CAD build for the part. Positions are in the model's coordinates, mm. Face numbers are marked on the shaded views. A direction names the side the tool comes from. Give positions to 0.01 mm unless a question says otherwise; leave off trailing zeros. Loops run counter-clockwise (first coordinate to the right, second up) from the corner with the lowest first, then second, coordinate; pieces in that order, holes last. Notation, with made-up numbers: M -9,45 L 50,45 A23 ccw 50,68 Z; hole C 35,70 d1. An arc over 180 degrees is marked long. Answer as CSV lines item,"result".
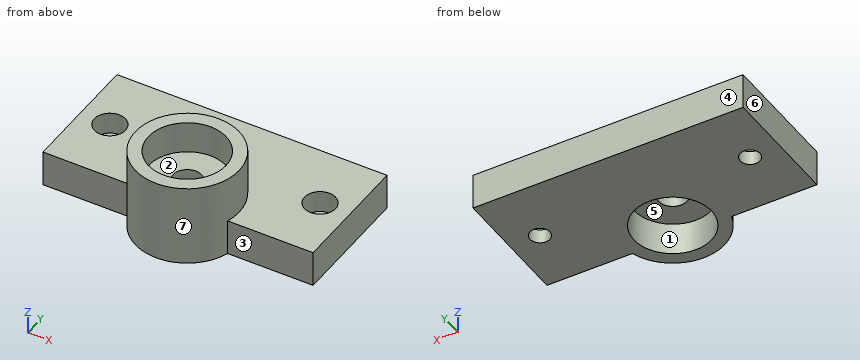
from build123d import *

# Parameters (mm, degrees)
F0_R     = 17.765
F0_R_2   = 13.28
F1_DEPTH = 27.96
F2_START = 11.06
F0_R_3   = 4.91
F2_DEPTH = 5.99
F3_R     = 5.32
F4_DEPTH = 12.28
F3_R_2   = 3.41
F5_DEPTH = 4.8


with BuildPart() as f1:
    # F0 (on Top) → F1 (new body)
    with BuildSketch(Plane.XY):
        Circle(F0_R)
        Circle(F0_R_2, mode=Mode.SUBTRACT)
    extrude(amount=F1_DEPTH)

    # F0 (on Top) → F2 (join)
    with BuildSketch(Plane.XY.offset(F2_START)):
        Circle(F0_R_2)
        Circle(F0_R_3, mode=Mode.SUBTRACT)
    extrude(amount=F2_DEPTH)

    # F3 (on Top) → F4 (join)
    with BuildSketch(Plane.XY):
        with BuildLine():
            Line((46.155, -5.28), (46.155, 37.06))
            Line((46.155, 37.06), (-46.155, 37.06))
            Line((-46.155, 37.06), (-46.155, -5.28))
            Line((-46.155, -5.28), (-12.1852369694, -5.28))
            ThreePointArc((-12.1852369694, -5.28), (-2.6961503154, 13.0034292968), (13.28, 0))
            ThreePointArc((13.28, 0), (13.0034292968, -2.6961503154), (12.1852369694, -5.28))
            Line((12.1852369694, -5.28), (46.155, -5.28))
        make_face()
        with Locations((-35.915, 15.87)):
            Circle(F3_R, mode=Mode.SUBTRACT)
        with Locations((35.915, 15.87)):
            Circle(F3_R, mode=Mode.SUBTRACT)
    extrude(amount=F4_DEPTH)

    # F3 (on Top) → F5 (join)
    with BuildSketch(Plane.XY):
        with Locations((-35.915, 15.87)):
            Circle(F3_R)
        with Locations((-35.915, 15.87)):
            Circle(F3_R_2, mode=Mode.SUBTRACT)
        with Locations((35.915, 15.87)):
            Circle(F3_R)
        with Locations((35.915, 15.87)):
            Circle(F3_R_2, mode=Mode.SUBTRACT)
    extrude(amount=F5_DEPTH)


solid = f1.part
1) Drill centre lines: line 1 (Y direction, x = 0, z = 4.75) (3 decimals); line 2 (Y direction, x = 0, z = 13.4) (3 decimals); line 3 (Y direction, x = 32, z = 3.25). Where is each one in solid material? Low to high. Write a range as from..to.
Answer below:
line 1,"y = -17.765..-13.28, 13.28..37.06"
line 2,"y = -17.765..-4.91, 4.91..17.765"
line 3,"y = -5.28..37.06"
2) Which spindle directions (+Z, -Z, +X, -X, +Y, -Y) get a long thin tool onto all of the face, cutting with end or side? Do the marked faces 1, 2 and 3. Say none if no direction does.
Answer below:
face 1,"-Z"
face 2,"+Z"
face 3,"+Z, -Z, +X, -Y"
3) Band-saw the part on B-B on y = 0. Give the cut face in (x, z) (3 decimals), and give its area (3 significant figures).
Answer below:
outline,"M -46.155,0 L -13.28,0 L -13.28,11.06 L -4.91,11.06 L -4.91,17.05 L -13.28,17.05 L -13.28,27.96 L -17.765,27.96 L -17.765,12.28 L -46.155,12.28 Z; M 4.91,11.06 L 13.28,11.06 L 13.28,0 L 46.155,0 L 46.155,12.28 L 17.765,12.28 L 17.765,27.96 L 13.28,27.96 L 13.28,17.05 L 4.91,17.05 Z"
area,"1,050 mm^2"
4) Band-saw the part on C-C on z = 7. Give the cut face in (x, y) (3 decimals).
Answer below:
outline,"M -46.155,-5.28 L -16.962,-5.28 A17.765 ccw 16.962,-5.28 L 46.155,-5.28 L 46.155,37.06 L -46.155,37.06 Z; hole C -35.915,15.87 d10.64; hole C 0,0 d26.56; hole C 35.915,15.87 d10.64"
5) Band-saw the part on D-D on y = 15.87. Give the cut face in (x, z) (3 decimals).
Answer below:
outline,"M -46.155,0 L -39.325,0 L -39.325,4.8 L -41.235,4.8 L -41.235,12.28 L -46.155,12.28 Z; M -32.505,0 L 32.505,0 L 32.505,4.8 L 30.595,4.8 L 30.595,12.28 L 7.984,12.28 L 7.984,27.96 L -7.984,27.96 L -7.984,12.28 L -30.595,12.28 L -30.595,4.8 L -32.505,4.8 Z; M 39.325,0 L 46.155,0 L 46.155,12.28 L 41.235,12.28 L 41.235,4.8 L 39.325,4.8 Z"
6) Band-saw the part on A-A on x = 0. Give the cut face in (y, z) (3 decimals).
Answer below:
outline,"M -17.765,0 L -13.28,0 L -13.28,11.06 L -4.91,11.06 L -4.91,17.05 L -13.28,17.05 L -13.28,27.96 L -17.765,27.96 Z; M 4.91,11.06 L 13.28,11.06 L 13.28,0 L 37.06,0 L 37.06,12.28 L 17.765,12.28 L 17.765,27.96 L 13.28,27.96 L 13.28,17.05 L 4.91,17.05 Z"
7) Mould opens along X. For the marked faces 4, 5, 6 and 7 say: +X half, -X half, draft (parallel to the pull), parting line (faces both ways), or undercut.
Answer below:
face 4,"draft"
face 5,"undercut"
face 6,"-X half"
face 7,"parting line"
8) Flat gauge pins, fed straight in: pin 1 (2 mm diameter, centred on y = -4.5, z = 16, fed in from -X); pin 2 (16 mm diameter, centred on x = 0, y = 0, fed in from +Z); pin 3 (1.5 mm diameter, centred on x = -29, y = 2.5, fed in from +Z); pin 4 (12 mm diameter, centred on x = -35.915, y = 15.87, fed in from -Z). Where does each tip first touch, or does it go through?
Answer below:
pin 1,"stops at x = -17.42"
pin 2,"stops at z = 17.05"
pin 3,"stops at z = 12.28"
pin 4,"stops at z = 0"
